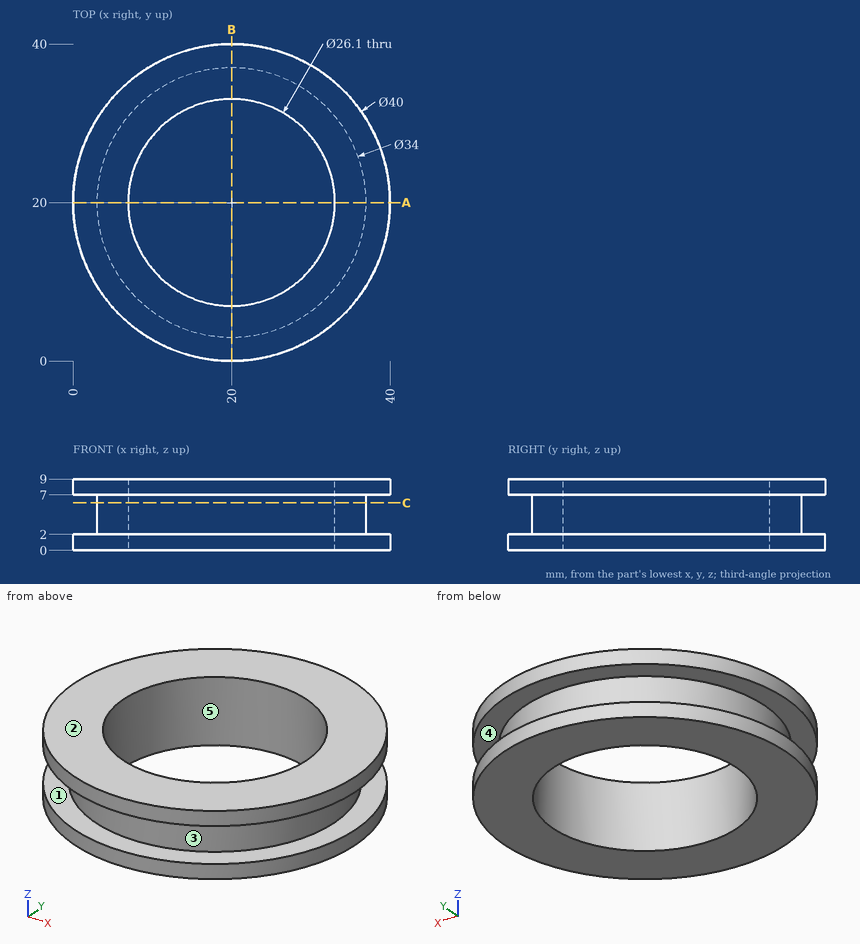
Verification items for this drawing (mm, ordinates from the low corner). A direction names the side the tool comes from. Coordinates: 2 decimals unless noted, no trailing zeros. Order: outer loops, then holes, each group sorted by start corner. A loop starts at its lowest first (then second) coordinate and runs counter-clockwise, first axis right, second up. Notation, with made-up numbers: (74.5, 64.25) -> (119.5, 64.25) arc R28 ccw to (119.5, 101.25) -> close; hole circle Ø6 at (28, 55). An arc over 180 degrees is marked (long way). Answer as CSV lines item,"result". Start each with the question number.
1) Set-up check for the marked faces 1 and 2: record each of +Z, -Z, +X, -X, +Y, -Y from which the full face is reachable in a straight line by a thin tool's end or side.
2) Cross-section at C-C, the plane z = 6. Record the boundary of the cut face in (x, y), then the cut area to 3 significant figures.
3) Cross-section at A-A, the plane y = 20. Record the boundary of the cut face in (x, z), then the cut area to 3 significant figures.
4) Material ranges on L1, parallel to Z at x = 36, y = 27.5; L2, parallel to Y at x = 20, z = 6.25; L3, parallel to Y at x = 20.5, z = 1.5, recorded low to high. Write a range as [from, to].
5) Release check for a two-part mould opening along Y. For the marked faces 3, 4 and 5 record: released by +Y, released by -Y, zero draft, split by the parting line, or undercut.
6) Gauge pin test, flat ends, axial feed: pin 1 Ø10 at (x, y) = (20.5, 23.5) entering from -Z; pin 2 Ø2 at (y, z) = (31, 7.5) entering from -X; pin 3 Ø4 at (x, z) = (17, 2.5) entering from +Y; pin 4 Ø20 at (x, y) = (16.5, 11) entering from +Z. Record the tip position at first contact, or that the pin passes through.
Conclusion:
1,face 1,"none"
1,face 2,"+Z, +X, -X, +Y, -Y"
2,outline,"circle Ø34 at (20, 20); hole circle Ø26.1 at (20, 20)"
2,area,"373 mm²"
3,outline,"(0, 0) -> (6.95, 0) -> (6.95, 9) -> (0, 9) -> (0, 7) -> (3, 7) -> (3, 2) -> (0, 2) -> close; (33.05, 0) -> (40, 0) -> (40, 2) -> (37, 2) -> (37, 7) -> (40, 7) -> (40, 9) -> (33.05, 9) -> close"
3,area,"95.1 mm²"
4,L1,"z = [0, 2], [7, 9]"
4,L2,"y = [3, 6.95], [33.05, 37]"
4,L3,"y = [0.01, 6.96], [33.04, 39.99]"
5,face 3,"split by the parting line"
5,face 4,"zero draft"
5,face 5,"undercut"
6,pin 1,"passes through"
6,pin 2,"stops at x = 2.68"
6,pin 3,"stops at y = 39.97"
6,pin 4,"stops at z = 9"
